from build123d import *

# Parameters (mm, degrees)
CUT_EXTRUDE1_DEPTH      = 58.948751496
CUT_EXTRUDE1_DEPTH_BACK = 58.948751496
CUT_EXTRUDE2_DEPTH      = 56.459898125
CIRPATTERN1_COUNT       = 7


with BuildPart() as part:
    # Sketch2 → Revolve3 (revolve)
    with BuildSketch(Plane(origin=(0, 0, 0), x_dir=(0, 0, -1), z_dir=(1, 0, 0)), mode=Mode.PRIVATE) as revolve3_sk:
        Polygon((12.7, 0), (12.7, 17.78), (6.35, 17.78), (6.35, 27.94), (12.7, 27.94), (12.7, 36.83), (9.525, 36.83), (6.35, 31.75), (-6.35, 31.75), (-9.525, 36.83), (-12.7, 36.83), (-12.7, 27.94), (-6.35, 27.94), (-6.35, 17.78), (-12.7, 17.78), (-12.7, 0), align=None)
    revolve(revolve3_sk.sketch.rotate(Axis((0, 0, 0), (0, 0, -1)), 90), axis=Axis((0, 0, 0), (0, 0, -1)))

    # Sketch3 → Cut-Extrude1 (cut, two sides: drawn at the far end of the back side and taken through both)
    with BuildSketch(Plane.XY.offset(12.7).offset(-CUT_EXTRUDE1_DEPTH_BACK)):
        with BuildLine():
            Line((-3.048, 12.065), (3.048, 12.065))
            Line((3.048, 12.065), (3.048, 9.024152093))
            ThreePointArc((3.048, 9.024152093), (0, -9.525), (-3.048, 9.024152093))
            Line((-3.048, 9.024152093), (-3.048, 12.065))
        make_face()
    extrude(amount=CUT_EXTRUDE1_DEPTH + CUT_EXTRUDE1_DEPTH_BACK, mode=Mode.SUBTRACT)

    # Sketch4 → Cut-Extrude2 (cut, through all)
    with BuildSketch(Plane.XY.offset(6.35)):
        with BuildLine():
            Line((-5.907465754, 22.046962339), (-5.413583315, 20.203767983))
            ThreePointArc((-5.413583315, 20.203767983), (-4.854909812, 19.452372744), (-3.933108575, 19.28807616))
            ThreePointArc((-3.933108575, 19.28807616), (0, 19.685), (3.933108575, 19.28807616))
            ThreePointArc((3.933108575, 19.28807616), (4.854909812, 19.452372744), (5.413583315, 20.203767983))
            Line((5.413583315, 20.203767983), (5.907465754, 22.046962339))
            ThreePointArc((5.907465754, 22.046962339), (5.762521779, 23.040980559), (4.940781063, 23.618754889))
            ThreePointArc((4.940781063, 23.618754889), (0, 24.13), (-4.940781063, 23.618754889))
            ThreePointArc((-4.940781063, 23.618754889), (-5.762521779, 23.040980559), (-5.907465754, 22.046962339))
        make_face()
    cut_extrude2 = extrude(amount=-CUT_EXTRUDE2_DEPTH, mode=Mode.SUBTRACT)

    # CirPattern1: Cut-Extrude2 ×7 about axis
    cirpattern1_axis = Axis((0, 0, 0), (0, 0, 1))
    for i in range(1, CIRPATTERN1_COUNT):
        add(cut_extrude2.rotate(cirpattern1_axis, i * 360 / CIRPATTERN1_COUNT), mode=Mode.SUBTRACT)


solid = part.part
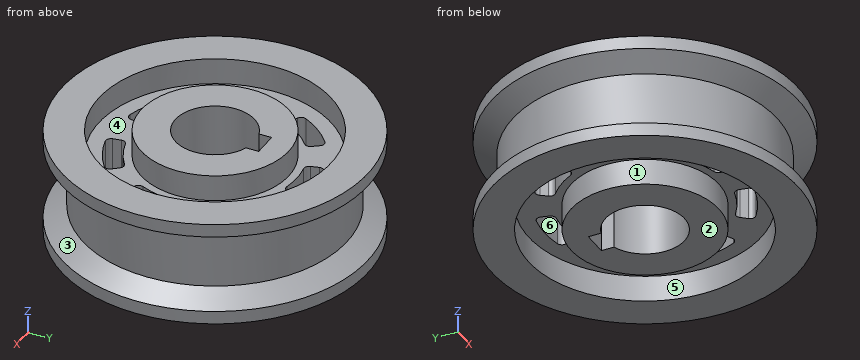
Model file for the job. Use its own axes, mm. Face numbers are marked on the shaded views. A direction names the side the tool comes from. Give positions to 0.01 mm unless a question says otherwise; leave off trailing zeros. Loops run counter-clockwise (first coordinate to the right, second up) from the corner with the lowest first, then second, coordinate; pieces in that order, holes last. Notation, with made-up numbers: (72, 33.25) -> (82, 33.25) arc R23 cw to (82, 62.25) -> close; hole circle Ø9 at (79, 21). An arc over 180 degrees is marked (long way). Use a Markdown table: item, result. Add a question column.
(1) Drop flat-ended pins along their axis: pin 1 Ø5 at (y, z) = (-17.5, -1) entering from -X; pin 2 Ø10 at (x, z) = (13, -0.5) entering from -Y; pin 3 Ø1.5 at (y, z) = (11.5, 1.5) entering from -X; pin 4 Ø15 at (x, y) = (0, 0) entering from +Z. Give the stop position or say it passes through.
(2) Slice it at A-A on z = -10.5. List the corners of the cut face in (x, y) (3 decimals), and give its area (3 significant figures).
(3) Tool access for the marked faces 4, 5 and 6: list every direction of +Z, -Z, +X, -X, +Y, -Y with a clear straight run to the whole face (end or side of a thin tool).
(4) Slice it at B-B on z = 7.75. List the corners of the cut face in (x, y) (3 decimals), and give its area (3 significant figures).
(5) Slice it at C-C on x = 0. Give the number of separate pieces and of enclosed holes in the cut face, and give its area (3 significant figures).
(6) Wall check: line 1 along X through (y, z) = (3.5, 11); line 2 along Y through (x, z) = (-18, 0); line 3 along Z through (x, y) = (33.5, -2). Give the ranges that are in metal, low to high.
(7) Mould opens along X. For the marked faces 1, 2 and 3 say: +X half, -X half, draft (parallel to the pull), parting line (faces both ways), or undercut.
Filled sheet:
| question | item | result |
|---|---|---|
| 1 | pin 1 | x = -27.98 |
| 1 | pin 2 | y = -30.73 |
| 1 | pin 3 | x = -29.87 |
| 1 | pin 4 | through |
| 2 | outline | circle Ø73.66 at (0, 0); circle Ø35.56 at (0, 0); hole circle Ø55.88 at (0, 0); hole (-3.048, 9.024) arc R9.525 ccw (long way) to (3.048, 9.024) -> (3.048, 12.065) -> (-3.048, 12.065) -> close |
| 2 | area | 2,500 mm2 |
| 3 | face 4 | +Z |
| 3 | face 5 | -Z |
| 3 | face 6 | +Z, -Z |
| 4 | outline | circle Ø67.98 at (0, 0); circle Ø35.56 at (0, 0); hole circle Ø55.88 at (0, 0); hole (-3.048, 9.024) arc R9.525 ccw (long way) to (3.048, 9.024) -> (3.048, 12.065) -> (-3.048, 12.065) -> close |
| 4 | area | 1,870 mm2 |
| 5 | separate pieces | 3 |
| 5 | enclosed holes | 0 |
| 5 | area | 847 mm2 |
| 6 | line 1 | -36.66 to -27.72, -17.43 to -8.86, 8.86 to 17.43, 27.72 to 36.66 |
| 6 | line 2 | -26.15 to -9.31, -7.97 to 8.45, 16.07 to 26.15 |
| 6 | line 3 | -12.7 to -7.48, 7.48 to 12.7 |
| 7 | face 1 | undercut |
| 7 | face 2 | draft |
| 7 | face 3 | parting line |
